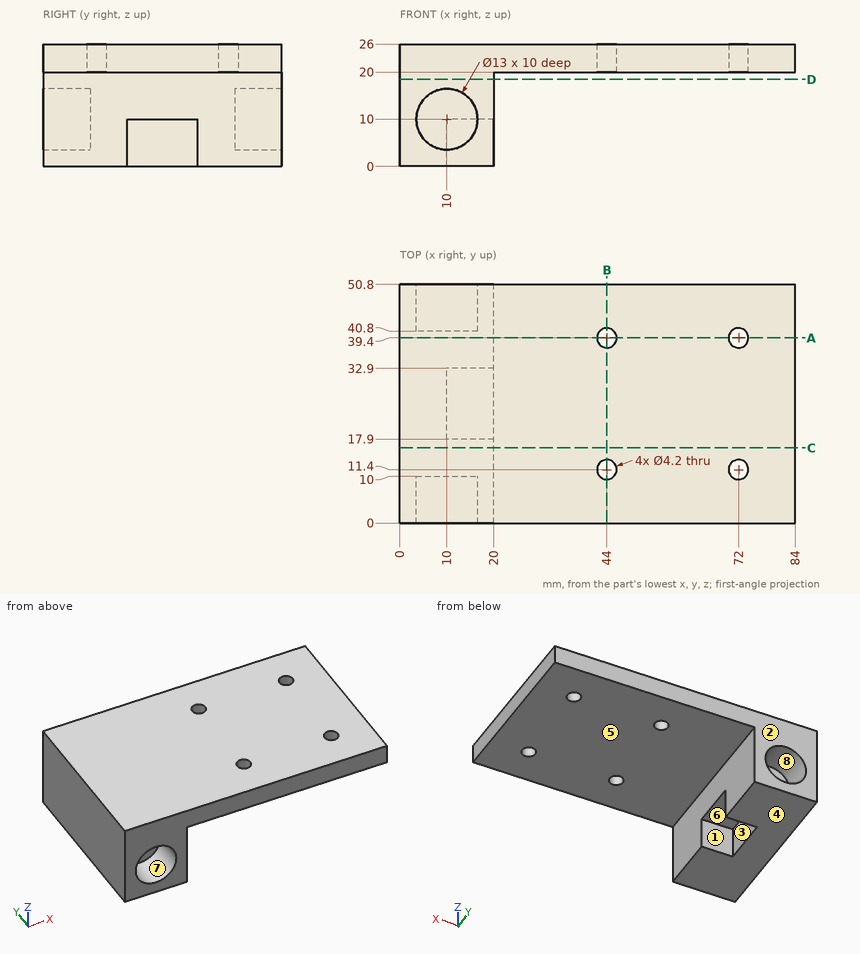
Source: three-view drawing plus pictorial views. Frame: mm from the lowest corner of the part. A direction names the side the tool comes from. Round coordinates to 2 decimals unless told otherwise and drop trailing zeros. Loops run counter-clockwise (first coordinate to the right, second up) from the corner with the lowest first, then second, coordinate; pieces in that order, holes last.
Q1. Section B-B, the plane x = 44. Return loops of the section in (y, z).
Q2. Access query for the marked faces 5, 6, 7 and 8. Directions: +Z, -Z, +X, -X, +Y, -Y. A direction counts if a zero-diameter tool reaches every point of the face in a straight line with its end or side. Return the directions, or none.
Q3. Section C-C, the plane y = 16. Return loops of the section in (x, z), plus the area to 3 significant figures.
Q4. Section D-D, the plane z = 18.5. Return loops of the section in (x, y).
Q5. Ray query, line 1 (Y direction, x = 44, z = 23.55); line 2 (X direction, y = 44.5, z = 9.5); line 3 (Z direction, x = 23.5, y = 33). Return the intervals inside material, ascending.
Q6. First-contact query: P1, Ø5, axis at x = 15, y = 29, coming from the -Z side; P2, Ø3.5, axis at x = 72, y = 39.4, coming from the +Z side; P3, Ø4, axis at x = 8.5, z = 10, coming from the -Y side; P4, Ø15, axis at x = 46, y = 19.5, coming from the -Z side. Flat tips, straight axial feed; report the tip coordinate or a pass-through.
Q7. Mould query, pull axis Y, two halves, no side actions, for the marked faces 1, 2, 3 and 4. Classes: pulls with the +Y half, pulls with the -Y half, needs draft (parallel to the pull), parting line crosses it, or undercut.
Q8. Section A-A, the plane y = 39.4. Return loops of the section in (x, z).
Solutions:
1. outline: (0, 20) - (9.3, 20) - (9.3, 26) - (0, 26) - close; (13.5, 20) - (37.3, 20) - (37.3, 26) - (13.5, 26) - close; (41.5, 20) - (50.8, 20) - (50.8, 26) - (41.5, 26) - close
2. face 5: -Z, +X, +Y, -Y
2. face 6: -Z, +X
2. face 7: -Y
2. face 8: +Y
3. outline: (0, 0) - (20, 0) - (20, 20) - (84, 20) - (84, 26) - (0, 26) - close
3. area: 904 mm2
4. outline: (0, 0) - (20, 0) - (20, 50.8) - (0, 50.8) - close
5. line 1: y = 0 to 9.3, 13.5 to 37.3, 41.5 to 50.8
5. line 2: x = 0 to 3.52, 16.48 to 20
5. line 3: z = 20 to 26
6. P1: stops at z = 10
6. P2: passes through
6. P3: stops at y = 10
6. P4: stops at z = 20
7. face 1: undercut
7. face 2: pulls with the +Y half
7. face 3: undercut
7. face 4: needs draft
8. outline: (0, 0) - (20, 0) - (20, 20) - (41.9, 20) - (41.9, 26) - (0, 26) - close; (46.1, 20) - (69.9, 20) - (69.9, 26) - (46.1, 26) - close; (74.1, 20) - (84, 20) - (84, 26) - (74.1, 26) - close
